Part model, mm, in its own coordinate system. Face numbers are marked on the shaded views. A direction names the side the tool comes from. Round coordinates to 2 decimals unless told otherwise and drop trailing zeros. Order: outer loops, then holes, each group sorted by start corner. A loop starts at its lowest first (then second) coordinate and runs counter-clockwise, first axis right, second up. Notation, with made-up numbers: (24.25, 52.5) - (74.25, 52.5) arc R5 ccw to (74.25, 57.5) - close; hole circle Ø10 at (31, -19.75). An arc over 180 degrees is marked (long way). Return JSON: item names as keys, results as strings. Group by question number.
Item 1: Saw through at D-D on y = 28. List the corners of the cut face in (x, z).
Item 2: Tool access for the marked faces 4, 5, 6, 7 and 8: list every direction of +Z, -Z, +X, -X, +Y, -Y with a clear straight run to the whole face (end or side of a thin tool).
Item 3: Saw through at B-B on x = 33. List the corners of the cut face in (y, z).
Item 4: Saw through at C-C on z = -4. List the corners of the cut face in (x, y), and give its area (3 significant figures).
Item 5: Probe probe 1 along Y at (x, z) = (42.5, -14.5); probe 2 along Z at (x, y) = (33, 1.75); probe 3 along X at (y, z) = (8.5, -8.5). List the from-to ranges inside material, lowest first.
Item 6: Saw through at A-A on y = 20.5. List the corners of the cut face in (x, z), and give its area (3 significant figures).
Item 7: Drop flat-ended pins along their axis: pin 1 (1.6 mm diameter, centred on y = 58.7, z = -4, fed in from -X); pin 2 (0.6 mm diameter, centred on x = 25, z = -0.5, fed in from +Y); pin 3 (3 mm diameter, centred on x = 16, z = -12, fed in from +Y); pin 4 (0.6 mm diameter, centred on x = 15, z = -29.5, fed in from -Y). Give the stop position or say it passes through.
Item 8: Two-plate mould, pull along Z, no slides. Class the marked faces 1, 2 and 3: released by +Z, released by -Z, zero draft, split by the parting line, or undercut.
```python
from build123d import *

# Parameters (mm, degrees)
SKETCH1_W            = 44
SKETCH1_H            = 30
BOSS_EXTRUDE1_DEPTH  = 54.5
SKETCH5_W            = 5
SKETCH5_H            = 30
BOSS_EXTRUDE3_DEPTH  = 6.8
SKETCH9_R            = 1.35
CUT_EXTRUDE6_DEPTH   = 6
FILLET1_R            = 1.5
FILLET2_R            = 1.25
SKETCH11_W           = 34
SKETCH11_H           = 26
CUT_EXTRUDE7_DEPTH   = 51.25
SKETCH13_R           = 5
SKETCH13_R_2         = 1.25
CUT_EXTRUDE8_DEPTH   = 3.25
CIRPATTERN1_COUNT    = 8
SKETCH15_W           = 20
SKETCH15_H           = 10
CUT_EXTRUDE10_DEPTH  = 5
FILLET6_R            = 1.5
FILLET6_OF_MIRROR4_R = 1.5
SKETCH16_W           = 34
SKETCH16_H           = 44.5
CUT_EXTRUDE11_DEPTH  = 2
FILLET7_R            = 1.25


with BuildPart() as part:
    # Sketch1 → Boss-Extrude1 (new body)
    with BuildSketch(Plane(origin=(0, 0, 0), x_dir=(1, 0, 0), z_dir=(0, 1, 0))):
        with Locations((22, 15)):
            Rectangle(SKETCH1_W, SKETCH1_H)
    extrude(amount=BOSS_EXTRUDE1_DEPTH)

    # Sketch5 → Boss-Extrude3 (add)
    with BuildSketch(Plane(origin=(0, 54.5, 0), x_dir=(1, 0, 0), z_dir=(0, 1, 0))):
        with Locations((2.5, 15)):
            Rectangle(SKETCH5_W, SKETCH5_H)
    boss_extrude3 = extrude(amount=BOSS_EXTRUDE3_DEPTH)

    # Sketch9 → Cut-Extrude6 (cut, through all)
    with BuildSketch(Plane(origin=(5, 0, 0), x_dir=(0, 0, -1), z_dir=(1, 0, 0))):
        with Locations((26, 58.7)):
            Circle(SKETCH9_R)
        with Locations((4, 58.7)):
            Circle(SKETCH9_R)
    cut_extrude6 = extrude(amount=-CUT_EXTRUDE6_DEPTH, mode=Mode.SUBTRACT)

    # Mirror2: Boss-Extrude3, Cut-Extrude6 across plane
    add(boss_extrude3.mirror(Plane.ZY.offset(-22)))
    add(cut_extrude6.mirror(Plane.ZY.offset(-22)), mode=Mode.SUBTRACT)

    # Fillet1
    fillet1_edges = [part.edges().sort_by_distance(p)[0] for p in [
        (2.5, 61.3, 0),
        (2.5, 61.3, -30),
        (41.5, 61.3, -30),
        (41.5, 61.3, 0),
    ]]
    fillet(fillet1_edges, radius=FILLET1_R)

    # Fillet2
    fillet2_edges = [part.edges().sort_by_distance(p)[0] for p in [
        (22, 0, -30),
        (44, 0, -15),
        (22, 0, 0),
        (0, 0, -15),
    ]]
    fillet(fillet2_edges, radius=FILLET2_R)

    # Sketch11 → Cut-Extrude7 (cut)
    with BuildSketch(Plane(origin=(0, 54.5, 0), x_dir=(1, 0, 0), z_dir=(0, 1, 0))):
        with Locations((22, 15)):
            Rectangle(SKETCH11_W, SKETCH11_H)
    extrude(amount=-CUT_EXTRUDE7_DEPTH, mode=Mode.SUBTRACT)

    # Sketch13 → Cut-Extrude8 (cut)
    with BuildSketch(Plane.XZ):
        with Locations((22, -15)):
            Circle(SKETCH13_R)
        with Locations((33, -15)):
            Circle(SKETCH13_R_2)
    cut_extrude8 = extrude(amount=-CUT_EXTRUDE8_DEPTH, mode=Mode.SUBTRACT)

    # CirPattern1: Cut-Extrude8 ×8 about axis
    cirpattern1_axis = Axis((22, 0, -15), (0, 1, 0))
    for i in range(1, CIRPATTERN1_COUNT):
        add(cut_extrude8.rotate(cirpattern1_axis, i * 360 / CIRPATTERN1_COUNT), mode=Mode.SUBTRACT)

    # Sketch15 → Cut-Extrude10 (cut)
    with BuildSketch(Plane(origin=(44, 0, 0), x_dir=(0, 0, -1), z_dir=(1, 0, 0))):
        with Locations((15, 18.25)):
            Rectangle(SKETCH15_W, SKETCH15_H)
        with Locations((15, 40.25)):
            Rectangle(SKETCH15_W, SKETCH15_H)
    cut_extrude10 = extrude(amount=-CUT_EXTRUDE10_DEPTH, mode=Mode.SUBTRACT)

    # Fillet6
    fillet6_edges = [part.edges().sort_by_distance(p)[0] for p in [
        (41.5, 23.25, -5),
        (41.5, 13.25, -5),
        (41.5, 13.25, -25),
        (41.5, 23.25, -25),
        (41.5, 45.25, -5),
        (41.5, 35.25, -5),
        (41.5, 35.25, -25),
        (41.5, 45.25, -25),
    ]]
    fillet(fillet6_edges, radius=FILLET6_R)

    # Mirror4: Cut-Extrude10 across plane
    add(cut_extrude10.mirror(Plane.ZY.offset(-22)), mode=Mode.SUBTRACT)

    # Fillet6 of Mirror4
    fillet6_of_mirror4_edges = [part.edges().sort_by_distance(p)[0] for p in [
        (2.5, 23.25, -5),
        (2.5, 13.25, -5),
        (2.5, 13.25, -25),
        (2.5, 23.25, -25),
        (2.5, 45.25, -5),
        (2.5, 35.25, -5),
        (2.5, 35.25, -25),
        (2.5, 45.25, -25),
    ]]
    fillet(fillet6_of_mirror4_edges, radius=FILLET6_OF_MIRROR4_R)

    # Sketch16 → Cut-Extrude11 (cut)
    with BuildSketch(Plane.XY):
        with Locations((22, 25.5)):
            Rectangle(SKETCH16_W, SKETCH16_H)
    cut_extrude11 = extrude(amount=-CUT_EXTRUDE11_DEPTH, mode=Mode.SUBTRACT)

    # Mirror5: Cut-Extrude11 across plane
    add(cut_extrude11.mirror(Plane(origin=(0, 0, -15), x_dir=(1, 0, 0), z_dir=(0, 0, -1))), mode=Mode.SUBTRACT)

    # Fillet7
    fillet7_edges = [part.edges().sort_by_distance(p)[0] for p in [
        (5, 54.5, -1),
        (5, 47.75, -1),
        (39, 47.75, -1),
        (5, 47.75, -29),
        (39, 47.75, -29),
        (39, 54.5, -1),
        (39, 54.5, -29),
        (5, 54.5, -29),
    ]]
    fillet(fillet7_edges, radius=FILLET7_R)


solid = part.part
```
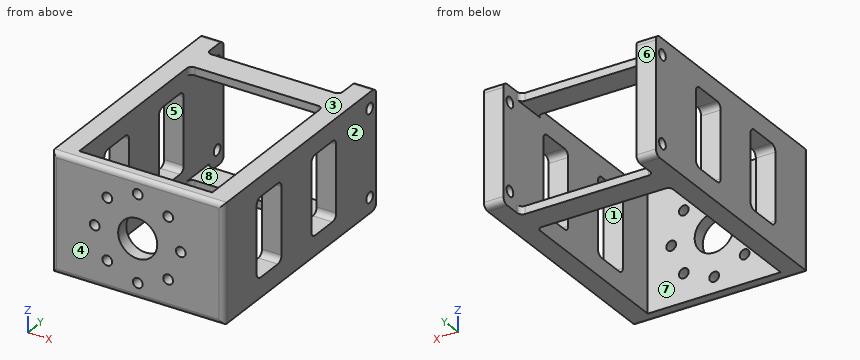
Filled in:
{
 "1": {"outline": "(0, -30) - (5, -30) - (5, 0) - (0, 0) - close; (39, -30) - (44, -30) - (44, 0) - (39, 0) - close"},
 "2": {"face 4": "+Z, -Z, +X, -X, -Y", "face 5": "+X, -X", "face 6": "+Z, -Z, +X, -X, +Y", "face 7": "+Z, -Z", "face 8": "+Y"},
 "3": {"outline": "(0, -28.75) arc R1.25 ccw to (1.25, -30) - (3.25, -30) - (3.25, -16.25) - (0, -16.25) - close; (0, -13.75) - (3.25, -13.75) - (3.25, 0) - (1.25, 0) arc R1.25 ccw to (0, -1.25) - close; (47.75, -30) - (54.5, -30) - (54.5, -28) - (47.75, -28) - close; (47.75, -2) - (54.5, -2) - (54.5, 0) - (47.75, 0) - close"},
 "4": {"outline": "(0, 1.25) arc R1.25 ccw to (1.25, 0) - (20.75, 0) - (20.75, 3.25) - (5, 3.25) - (5, 57.35) - (0, 57.35) - close; (0, 60.05) - (5, 60.05) - (5, 61.3) - (0, 61.3) - close; (23.25, 0) - (42.75, 0) arc R1.25 ccw to (44, 1.25) - (44, 57.35) - (39, 57.35) - (39, 3.25) - (23.25, 3.25) - close; (39, 60.05) - (44, 60.05) - (44, 61.3) - (39, 61.3) - close", "area": "688 mm^2"},
 "5": {"probe 1": "y = 0 to 13.25, 23.25 to 35.25, 45.25 to 61.3", "probe 2": "z = -30 to -16.25, -13.75 to 0", "probe 3": "x = 0 to 5, 39 to 44"},
 "6": {"outline": "(0, -30) - (5, -30) - (5, -25) - (0, -25) - close; (0, -5) - (5, -5) - (5, 0) - (0, 0) - close; (39, -30) - (44, -30) - (44, -25) - (39, -25) - close; (39, -5) - (44, -5) - (44, 0) - (39, 0) - close", "area": "100 mm^2"},
 "7": {"pin 1": "passes through", "pin 2": "stops at y = 54.5", "pin 3": "stops at y = 3.25", "pin 4": "stops at y = 0.08"},
 "8": {"face 1": "undercut", "face 2": "zero draft", "face 3": "released by +Z"}
}
